Work out the finished part from the listing and answer in its coordinate system (mm). Coordinates: 2 decimals unless noted, no trailing zeros. Order: outer loops, then holes, each group sorted by start corner. A loop starts at its lowest first (then second) coordinate and runs counter-clockwise, first axis right, second up. Notation, with made-up numbers: M 37,-30.5 L 74,-30.5 A35 ccw 74,8.5 Z; hole C 66,-23.5 d6. An arc over 180 degrees is marked long. Use a Markdown table: item, result. Add a question column.
from build123d import *

# Parameters (mm, degrees)
SKETCH1_R             = 4.953
BOSS_EXTRUDE1_DEPTH   = 50.8
BOSS_EXTRUDE2_START   = -3.81
SKETCH2_R             = 5.3975
SKETCH2_R_2           = 4.953
BOSS_EXTRUDE2_DEPTH   = 3.81
F_4_40_TAPPED_HOLE1_D = 2.2606


with BuildPart() as part:
    # Sketch1 → Boss-Extrude1 (new body)
    with BuildSketch(Plane(origin=(0, 0, 0), x_dir=(1, 0, 0), z_dir=(0, 1, 0))):
        with Locations(Location((0, 0, 0), (0, 0, 270))):
            Circle(SKETCH1_R)
    extrude(amount=BOSS_EXTRUDE1_DEPTH)

    # Sketch2 → Boss-Extrude2 (add)
    with BuildSketch(Plane(origin=(0, 50.8, 0), x_dir=(1, 0, 0), z_dir=(0, 1, 0)).offset(BOSS_EXTRUDE2_START)):
        with Locations(Location((0, 0, 0), (0, 0, 270))):
            Circle(SKETCH2_R)
        with Locations(Location((0, 0, 0), (0, 0, 270))):
            Circle(SKETCH2_R_2, mode=Mode.SUBTRACT)
    extrude(amount=BOSS_EXTRUDE2_DEPTH)

    # #4-40 Tapped Hole1 (through all)
    with Locations(Plane.XY.offset(4.953)):
        with Locations((0, 5.08)):
            Hole(F_4_40_TAPPED_HOLE1_D / 2)


solid = part.part
(1) Straight lines are drawn through the part: line 1 (Y direction, x = 0, z = 0.25); line 2 (X direction, y = 5.08, z = 1); line 3 (Y direction, x = -0.75, z = -2.5). For each, find the intervals that lie inside material, in ascending order.
(2) A cutting plane is placed at A-A on x = 0. Write down the section's boundary in (y, z), plus the area to 3 significant figures.
(3) A cutting plane is placed at B-B on z = 0. Write down the section's boundary in (x, y).
(4) A cutting plane is placed at C-C on y = 5.08. Write down the section's boundary in (x, z).
(5) A cutting plane is placed at D-D on x = -2.5. Write down the section's boundary in (y, z), plus the area to 3 significant figures.
(6) The mould has two halves that part along Y. Classify faces 1 (the flat face through (0, 0, 0)), 2 (the flat face through (0, 50.8, 0)), 3 (the cylindrical face through (3.648, 48.868, -3.978)), 4 (the cylindrical face through (-0.61, 6.03, -0.07)): pulls with the +Y half, pulls with the -Y half, needs draft (parallel to the pull), parting line crosses it, or undercut.
(7) Given P1, Ø2.5, axis at x = 0, y = 5.08, coming from the +Z side; P2, Ø4, axis at x = 3.5, y = 12, coming from the -Z side; P3, Ø1, axis at y = 5, z = -4, coming from the -X side, each flat-ended and moving along its own axis, determine where each tip first touches the part or whether it passes through.
From the geometry:
| question | item | result |
|---|---|---|
| 1 | line 1 | y = 0 to 3.95, 6.21 to 50.8 |
| 1 | line 2 | x = -4.85 to -1.13, 1.13 to 4.85 |
| 1 | line 3 | y = 0 to 4.23, 5.93 to 50.8 |
| 2 | outline | M 0,-4.95 L 3.95,-4.95 L 3.95,4.95 L 0,4.95 Z; M 6.21,-4.95 L 46.99,-4.95 L 46.99,-5.4 L 50.8,-5.4 L 50.8,5.4 L 46.99,5.4 L 46.99,4.95 L 6.21,4.95 Z |
| 2 | area | 484 mm2 |
| 3 | outline | M -5.4,46.99 L -4.95,46.99 L -4.95,0 L 4.95,0 L 4.95,46.99 L 5.4,46.99 L 5.4,50.8 L -5.4,50.8 Z; hole C 0,5.08 d2.26 |
| 4 | outline | M -1.13,-4.82 L -1.13,4.82 A4.95 ccw Z; M 1.13,-4.82 A4.95 ccw 1.13,4.82 Z |
| 5 | outline | M 0,-4.28 L 46.99,-4.28 L 46.99,-4.78 L 50.8,-4.78 L 50.8,4.78 L 46.99,4.78 L 46.99,4.28 L 0,4.28 Z |
| 5 | area | 438 mm2 |
| 6 | face 1 | pulls with the -Y half |
| 6 | face 2 | pulls with the +Y half |
| 6 | face 3 | needs draft |
| 6 | face 4 | undercut |
| 7 | P1 | stops at z = 4.95 |
| 7 | P2 | stops at z = -4.72 |
| 7 | P3 | stops at x = -3.5 |
